Geometry check sheet. Reference: the model listing, model coordinates, mm. A direction names the side the tool comes from. Give positions to 0.01 mm unless a question says otherwise; leave off trailing zeros. Order: outer loops, then holes, each group sorted by start corner. A loop starts at its lowest first (then second) coordinate and runs counter-clockwise, first axis right, second up. Notation, with made-up numbers: M -6.75,-22.5 L 48.25,-22.5 A29 ccw 48.25,-2.5 Z; hole C 4,17 d3. An arc over 180 degrees is marked long. Answer as CSV lines item,"result".
from build123d import *

# Parameters (mm, degrees)
SKETCH1_R           = 1.5
SKETCH1_R_2         = 0.75
BOSS_EXTRUDE1_DEPTH = 3.125
SKETCH2_W           = 0.5
SKETCH2_H           = 3
BOSS_EXTRUDE2_DEPTH = 4


with BuildPart() as part:
    # Sketch1 → Boss-Extrude1 (new body, symmetric)
    with BuildSketch(Plane.XY):
        Polygon((10, 0), (-10, 0), (-10, 10), (-1, 10), (-0.133974596, 9.5), (10, 9.5), align=None)
        with Locations((-5, 2.5)):
            Circle(SKETCH1_R, mode=Mode.SUBTRACT)
        with Locations((5, 2.5)):
            Circle(SKETCH1_R, mode=Mode.SUBTRACT)
        with Locations((-7, 8.5)):
            Circle(SKETCH1_R_2, mode=Mode.SUBTRACT)
    extrude(amount=BOSS_EXTRUDE1_DEPTH, both=True)

    # Sketch2 → Boss-Extrude2 (add)
    with BuildSketch(Plane.XZ):
        Rectangle(SKETCH2_W, SKETCH2_H)
        with Locations((-8, 0)):
            Rectangle(SKETCH2_W, SKETCH2_H)
        with Locations((8, 0)):
            Rectangle(SKETCH2_W, SKETCH2_H)
    extrude(amount=BOSS_EXTRUDE2_DEPTH)


solid = part.part
(1) Gauge pin test, flat ends, axial feed: P1, Ø0.6, axis at x = 8, y = -2.5, coming from the +Z side; P2, Ø1.5, axis at x = 5, z = 1, coming from the -Y side; P3, Ø2.5, axis at y = -1.5, z = 0.5, coming from the +X side. Record the tip position at first contact, or that the pin passes through.
The answers:
P1,"stops at z = 1.5"
P2,"stops at y = 0"
P3,"stops at x = 8.25"
(2) Material ranges on line 1 (Y direction, x = 5, z = -2); line 2 (Y direction, x = -7, z = 0); line 3 (X direction, y = 1.75, z = -0.5), recorded low to high.
The answers:
line 1,"y = 0 to 1, 4 to 9.5"
line 2,"y = 0 to 7.75, 9.25 to 10"
line 3,"x = -10 to -6.3, -3.7 to 3.7, 6.3 to 10"
(3) Section check C-C on z = 0.75. Enter the section's corners in (x, y).
The answers:
outline,"M -10,0 L -8.25,0 L -8.25,-4 L -7.75,-4 L -7.75,0 L -0.25,0 L -0.25,-4 L 0.25,-4 L 0.25,0 L 7.75,0 L 7.75,-4 L 8.25,-4 L 8.25,0 L 10,0 L 10,9.5 L -0.13,9.5 L -1,10 L -10,10 Z; hole C -7,8.5 d1.5; hole C -5,2.5 d3; hole C 5,2.5 d3"
(4) Tool access check on faces 1 (the face through (-8.25, -2, 0)), 2 (the face through (0.25, -2, 0)), 3 (the face through (-7.55, 9.01, -0.04)). Record the directions out of +Z, -Z, +X, -X, +Y, -Y that give a thin tool (end or side, any length) a straight path to the whole face; none if there is none.
The answers:
face 1,"+Z, -Z, -X, -Y"
face 2,"+Z, -Z, -Y"
face 3,"+Z, -Z"
(5) Section check B-B on y = 2.5. Enter the section's corners in (x, z) (3 decimals), then the cut area to 3 significant figures.
The answers:
outline,"M -10,-3.125 L -6.5,-3.125 L -6.5,3.125 L -10,3.125 Z; M -3.5,-3.125 L 3.5,-3.125 L 3.5,3.125 L -3.5,3.125 Z; M 6.5,-3.125 L 10,-3.125 L 10,3.125 L 6.5,3.125 Z"
area,"87.5 mm2"
(6) Section check A-A on x = -5. Enter the section's corners in (y, z) (3 decimals), then the cut area to 4 significant figures.
The answers:
outline,"M 0,-3.125 L 1,-3.125 L 1,3.125 L 0,3.125 Z; M 4,-3.125 L 10,-3.125 L 10,3.125 L 4,3.125 Z"
area,"43.75 mm2"
(7) Draft check along Y on faces 4 (the face through (5.69, 1.17, -0.04)), 5 (the face through (5, 9.5, 0)), 6 (the face through (8.25, -2, 0)). Enter one of: +Y half, -Y half, draft (parallel to the pull), parting line (faces both ways), or undercut.
The answers:
face 4,"undercut"
face 5,"+Y half"
face 6,"draft"
(8) Section check D-D on x = 5. Enter the section's corners in (y, z) (3 decimals), then the cut area to 3 significant figures.
The answers:
outline,"M 0,-3.125 L 1,-3.125 L 1,3.125 L 0,3.125 Z; M 4,-3.125 L 9.5,-3.125 L 9.5,3.125 L 4,3.125 Z"
area,"40.6 mm2"
